Here's the drawing with two shaded views (mm, measured from the low corner). I have some questions. A direction names the side the tool comes from. Coordinates: 2 decimals unless noted, no trailing zeros. Write each loop counter-clockwise with the first axis right and the second up, starting at its lowest first coordinate (ties: lowest second). Pieces come first, ordered by that corner, then holes.
Item 1: Thinking about a two-plate mould opening in Y: for the marked faces 3, 4 and 5, which applies, +Y half, -Y half, draft (parallel to the pull), parting line (faces both ways), or undercut?
Item 2: Which directions (+Z, -Z, +X, -X, +Y, -Y) give clear straight access to the entire face, cutting with the end or side of a thin tool? Please do the marked faces 1 and 2.
Item 3: For P1, Ø5, axis at x = 55.5, y = 9, coming from the -Z side; P2, Ø12.5, axis at x = 25.5, y = 14.5, coming from the -Z side; P3, Ø3, axis at x = 40.5, y = 12, coming from the -Z side, each with a flat end and sliding along its axis, tell me the tip position at first contact or that it passes through.
Item 4: I want a section at A-A on z = 51. Please give me the cut outline in (x, y) (1 decimal), then the cut area to 3 significant figures.
Item 5: I want a section at C-C on x = 70. Please give me the cut outline in (y, z), then the cut area to 3 significant figures.
Item 6: I want a section at B-B on z = 20.5. Please give me the cut outline in (x, y).
Item 7: If I drill on probe 1 along Z at (x, y) = (44, 11.75); probe 2 along Z at (x, y) = (78, 18.25); probe 3 along X at (y, z) = (12.75, 20) (1 decimal), over which ranges is the centre line in solid material (lowest first)?
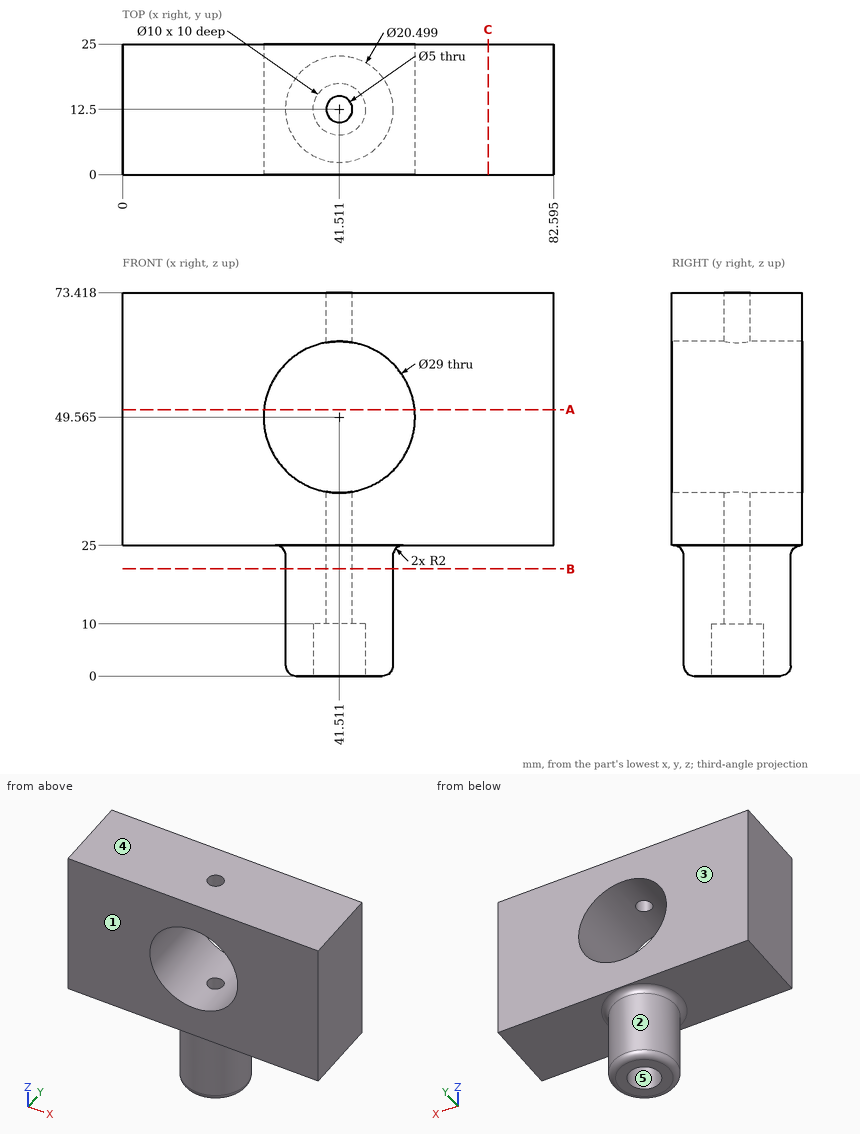
Response values:
1. face 3: +Y half
1. face 4: draft
1. face 5: undercut
2. face 1: +Z, -Z, +X, -X, -Y
2. face 2: -Z
3. P1: stops at z = 24.97
3. P2: stops at z = 0.85
3. P3: stops at z = 10
4. outline: (0, 0) - (27.1, 0) - (27.1, 25) - (0, 25) - close; (55.9, 0) - (82.6, 0) - (82.6, 25) - (55.9, 25) - close
4. area: 1,340 mm2
5. outline: (0, 25) - (25, 25) - (25, 73.42) - (0, 73.42) - close
5. area: 1,210 mm2
6. outline: circle Ø20.5 at (41.51, 12.5); hole circle Ø5 at (41.51, 12.5)
7. probe 1: z = 10 to 35.28, 63.85 to 73.42
7. probe 2: z = 25 to 73.42
7. probe 3: x = 31.3 to 39, 44 to 51.8
